Part model, mm, in its own coordinate system. A direction names the side the tool comes from. Coordinates: 2 decimals unless noted, no trailing zeros. Order: outer loops, then holes, each group sorted by start corner. A loop starts at its lowest first (then second) coordinate and runs counter-clockwise, first axis right, second up. Notation, with made-up numbers: (28.5, -39) - (71.5, -39) arc R5 ccw to (71.5, -34) - close; hole circle Ø9 at (75.5, -23.5). An arc over 180 degrees is marked (long way). Use a Markdown table: item, result. Add a question column.
1) Wall check: L1, parallel to Z at x = 8.5, y = -3.5; L2, parallel to X at y = -4, z = -17; L3, parallel to X at y = -4, z = 33. Give the ranges that are in metal, low to high. Write a range as [from, to].
2) Saw through at B-B on z = -27.5. List the corners of the cut face in (x, y), then the cut area to 3 significant figures.
3) Two-plate mould, pull along X, no slides. Class faces 1 (the face through (0.287, -3.451, 55.866)), 2 (the face through (-32.964, -3.451, -15.671)), 3 (the face through (16.236, -3.451, 8.828)), 4 (the face through (0, -7, -12)): +X half, -X half, draft (parallel to the pull), parting line (faces both ways), or undercut.
4) Drop flat-ended pins along their axis: P1, Ø3.5, axis at y = -4.5, z = 47, coming from the +X side; P2, Ø13, axis at x = 0, z = 0, coming from the +Y side (3 decimals); P3, Ø4, axis at x = -29.5, y = -6, coming from the -Z side; P4, Ø2, axis at y = -4, z = 43.5, coming from the -X side. Give the stop position or say it passes through.
5) Saw through at A-A on z = 44.45. List the corners of the cut face in (x, y) (3 decimals).
6) Tool access for faces 5 (the face through (-15.76, -3.45, 9.65)), 6 (the face through (-8.575, -3, 44)): list every direction of +Z, -Z, +X, -X, +Y, -Y with a clear straight run to the whole face (end or side of a thin tool).
7) Saw through at D-D on z = -8. List the corners of the cut face in (x, y), then the cut area to 3 significant figures.
8) Saw through at C-C on y = -3.25. Count the separate pieces of the cut face and the enclosed holes in it, then the cut area to 3 significant figures.
```python
from build123d import *

# Parameters (mm, degrees)
F0_R     = 10.9
F1_DEPTH = 7


with BuildPart() as f1:
    # F0 (on Front) → F1 (new body)
    with BuildSketch(Plane.XZ):
        with BuildLine():
            ThreePointArc((41.8292028353, -11.3029487912), (15.9973702481, 9.2360860191), (11.1259606268, 41.876626671))
            ThreePointArc((11.1259606268, 41.876626671), (0, 55.8696869554), (-11.1259606268, 41.876626671))
            ThreePointArc((-11.1259606268, 41.876626671), (-15.9973702481, 9.2360860191), (-41.8292028353, -11.3029487912))
            ThreePointArc((-41.8292028353, -11.3029487912), (-48.3845682049, -27.9348434777), (-30.7032422085, -30.5736778798))
            ThreePointArc((-30.7032422085, -30.5736778798), (0, -18.4721720382), (30.7032422085, -30.5736778798))
            ThreePointArc((30.7032422085, -30.5736778798), (48.3845682049, -27.9348434777), (41.8292028353, -11.3029487912))
        make_face()
        Polygon((-36.6695744207, -12.4931307895), (-29.1541558468, -18.9397824005), (-30.9794106244, -28.671651611), (-33.2699969614, -29.4772760306), (-40.3200839758, -31.9568692105), (-47.8355025496, -25.5102175995), (-46.010247772, -15.778348389), (-42.056981042, -14.3879409796), align=None, mode=Mode.SUBTRACT)
        Polygon((42.294572947, -13.6737558569), (48.1637383341, -20.0912171021), (45.1771939619, -29.5316294896), (35.508284826, -31.6654123875), (33.3864310519, -29.3453356023), (28.8259200623, -24.3587828979), (31.8124644346, -14.9183705104), (41.4813735704, -12.7845876125), align=None, mode=Mode.SUBTRACT)
        Circle(F0_R, mode=Mode.SUBTRACT)
        Polygon((0, 54.3515571166), (8.575, 49.4007785583), (8.575, 43.6150418434), (8.575, 39.4992214417), (0, 34.5484428834), (-8.575, 39.4992214417), (-8.575, 43.6150418434), (-8.575, 49.4007785583), align=None, mode=Mode.SUBTRACT)
    extrude(amount=F1_DEPTH)


solid = f1.part
```
Results are:
| question | item | result |
|---|---|---|
| 1 | L1 | [-19.28, -6.82], [6.82, 39.46], [49.44, 52.08] |
| 1 | L2 | [-48.65, -46.24], [-31.42, 31.15], [45.34, 48.65] |
| 1 | L3 | [-9.99, 9.99] |
| 2 | outline | (-48.62, -7) - (-45.52, -7) - (-45.52, 0) - (-48.62, 0) - close; (-30.76, -7) - (-27.04, -7) - (-27.04, 0) - (-30.76, 0) - close; (27.04, -7) - (31.7, -7) - (31.7, 0) - (27.04, 0) - close; (45.82, -7) - (48.62, -7) - (48.62, 0) - (45.82, 0) - close |
| 2 | area | 100 mm2 |
| 3 | face 1 | parting line |
| 3 | face 2 | undercut |
| 3 | face 3 | +X half |
| 3 | face 4 | draft |
| 4 | P1 | x = 11.39 |
| 4 | P2 | through |
| 4 | P3 | z = -31.25 |
| 4 | P4 | x = -11.42 |
| 5 | outline | (-11.42, -7) - (-8.575, -7) - (-8.575, 0) - (-11.42, 0) - close; (8.575, -7) - (11.42, -7) - (11.42, 0) - (8.575, 0) - close |
| 6 | face 5 | -X, +Y, -Y |
| 6 | face 6 | +Y, -Y |
| 7 | outline | (-33.85, -7) - (-7.4, -7) - (-7.4, 0) - (-33.85, 0) - close; (7.4, -7) - (33.85, -7) - (33.85, 0) - (7.4, 0) - close |
| 7 | area | 370 mm2 |
| 8 | separate pieces | 1 |
| 8 | enclosed holes | 4 |
| 8 | area | 2,330 mm2 |
